```python
from build123d import *

# Parameters (mm, degrees)
SKETCH1_R           = 8.05
BOSS_EXTRUDE1_DEPTH = 11.15
SKETCH2_R           = 3.175
F_25_HOLE_DEPTH     = 7.4
SKETCH3_R           = 2.54
F_0_2_HOLE_DEPTH    = 7.4


with BuildPart() as part:
    # Sketch1 → Boss-Extrude1 (new body, symmetric)
    with BuildSketch(Plane(origin=(0, 0, 0), x_dir=(1, 0, 0), z_dir=(0, 1, 0))):
        Circle(SKETCH1_R)
    extrude(amount=BOSS_EXTRUDE1_DEPTH, both=True)

    # Sketch2 → .25" hole (cut)
    with BuildSketch(Plane(origin=(0, 11.15, 0), x_dir=(1, 0, 0), z_dir=(0, 1, 0))):
        Circle(SKETCH2_R)
    extrude(amount=-F_25_HOLE_DEPTH, mode=Mode.SUBTRACT)

    # Sketch3 → 0.2" hole (cut)
    with BuildSketch(Plane.XZ.offset(11.15)):
        Circle(SKETCH3_R)
    extrude(amount=-F_0_2_HOLE_DEPTH, mode=Mode.SUBTRACT)


solid = part.part
```
Model file for the job. Use its own axes, mm. A direction names the side the tool comes from. Coordinates: 2 decimals unless noted, no trailing zeros. Write each loop counter-clockwise with the first axis right and the second up, starting at its lowest first coordinate (ties: lowest second). Pieces come first, ordered by that corner, then holes. Notation, with made-up numbers: (-40, 9.5) - (-25, 9.5) arc R15 cw to (-25, 19.5) - close; hole circle Ø6 at (-23, 12.25). An arc over 180 degrees is marked (long way). One line per item, written item: value. Start each with the question number.
1. Slice it at C-C (y = -5.75). Write the cut outline in (x, z), plus the area to 3 significant figures.
2. Slice it at D-D (y = -3). Write the cut outline in (x, z).
3. Tool access for faces 4 (the flat face through (-2, -11.15, -2)), 5 (the flat face through (0, -3.75, 0)), 6 (the flat face through (0, 3.75, 0)): list every direction of +Z, -Z, +X, -X, +Y, -Y with a clear straight run to the whole face (end or side of a thin tool).
4. Mould opens along X. For faces 1 (the flat face through (3.5, 11.15, -0.1)), 2 (the cylindrical face through (-0.33, -7.5, 2.52)), 3 (the cylindrical face through (7.678, 0.156, -2.418)) say: released by +X, released by -X, zero draft, split by the parting line, or undercut.
5. Slice it at A-A (x = 0). Write the cut outline in (y, z) (3 decimals).
6. Slice it at B-B (z = 0). Write the cut outline in (x, y) (3 decimals), plus the area to 3 significant figures.
7. Probe line 1 (Z direction, x = 0, y = 7.75) (3 decimals); line 2 (Z direction, x = 0, y = -5.25); line 3 (Y direction, x = -0.5, z = -1.75). List the from-to ranges inside material, lowest first. Write a range as from..to.
8. Flat gauge pins, fed straight in: pin 1 (1 mm diameter, centred on x = -2.5, y = 2.5, fed in from -Z); pin 2 (1.5 mm diameter, centred on x = -5, y = 6, fed in from +Z); pin 3 (2 mm diameter, centred on y = 7, z = -3, fed in from +X). Where does each tip first touch, or does it go through?
Answers below:
1. outline: circle Ø16.1 at (0, 0); hole circle Ø5.08 at (0, 0)
1. area: 183 mm^2
2. outline: circle Ø16.1 at (0, 0)
3. face 4: +Z, -Z, +X, -X, -Y
3. face 5: -Y
3. face 6: +Y
4. face 1: zero draft
4. face 2: undercut
4. face 3: split by the parting line
5. outline: (-11.15, -8.05) - (11.15, -8.05) - (11.15, -3.175) - (3.75, -3.175) - (3.75, 3.175) - (11.15, 3.175) - (11.15, 8.05) - (-11.15, 8.05) - (-11.15, 2.54) - (-3.75, 2.54) - (-3.75, -2.54) - (-11.15, -2.54) - close
6. outline: (-8.05, -11.15) - (-2.54, -11.15) - (-2.54, -3.75) - (2.54, -3.75) - (2.54, -11.15) - (8.05, -11.15) - (8.05, 11.15) - (3.175, 11.15) - (3.175, 3.75) - (-3.175, 3.75) - (-3.175, 11.15) - (-8.05, 11.15) - close
6. area: 274 mm^2
7. line 1: z = -8.05..-3.175, 3.175..8.05
7. line 2: z = -8.05..-2.54, 2.54..8.05
7. line 3: y = -3.75..3.75
8. pin 1: stops at z = -7.8
8. pin 2: stops at z = 6.84
8. pin 3: stops at x = 7.8
